Input: dimensioned drawing with shaded views. Units: mm. Origin: part minimum x, y, z. Give positions to 0.01 mm unless a question says otherwise; leave off trailing zeros. Write each loop counter-clockwise with the first axis right and the second up, starting at its lowest first coordinate (ties: lowest second). Pieces come first, ordered by that corner, then holes.
Q1. Section B-B (z = 25). Return the cut outline in (x, y), plus the area to 3 significant figures.
Q2. Line query: line 1 (Z direction, x = 190, y = 1.6); line 2 (X direction, y = 1.65, z = 16); line 3 (Z direction, x = 127, y = 1.45). Output: solid intervals per line, ascending.
Q3. Pin query (flat end, axial travel): pin 1 Ø2.5 at (x, z) = (160, 21.25) entering from -Y. Return the tip coordinate at first contact, or that it passes through.
Q4. Section A-A (y = 0.8). Return the cut outline in (x, z).
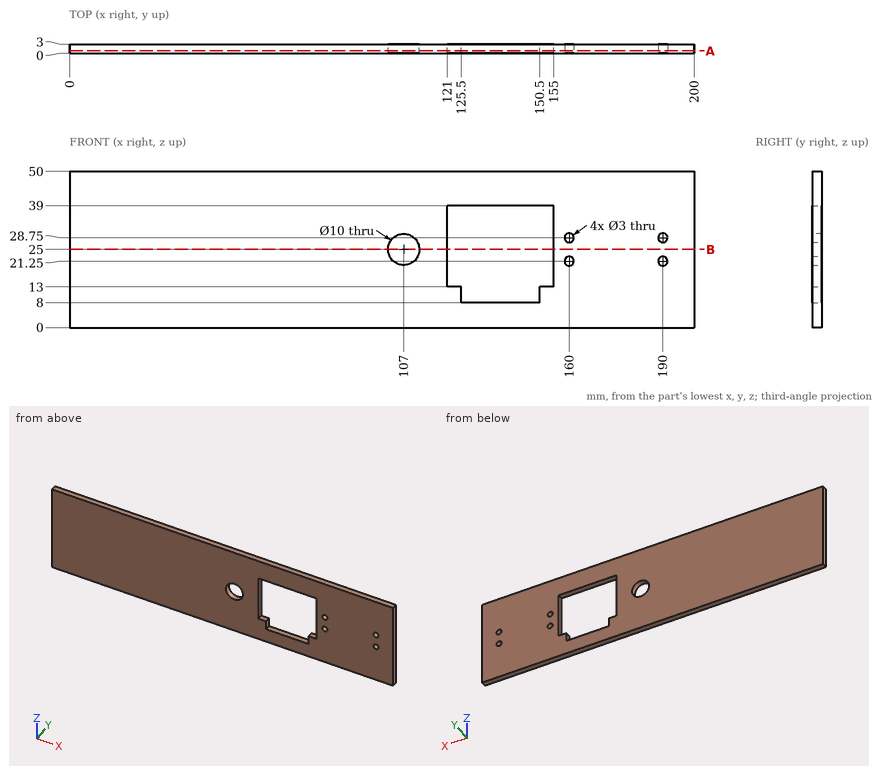
Computed:
1. outline: (0, 0) - (102, 0) - (102, 3) - (0, 3) - close; (112, 0) - (121, 0) - (121, 3) - (112, 3) - close; (155, 0) - (200, 0) - (200, 3) - (155, 3) - close
1. area: 468 mm2
2. line 1: z = 0 to 19.75, 22.75 to 27.25, 30.25 to 50
2. line 2: x = 0 to 121, 155 to 200
2. line 3: z = 0 to 8, 39 to 50
3. pin 1: passes through
4. outline: (0, 0) - (200, 0) - (200, 50) - (0, 50) - close; hole circle Ø10 at (107, 25); hole (121, 13) - (125.5, 13) - (125.5, 8) - (150.5, 8) - (150.5, 13) - (155, 13) - (155, 39) - (121, 39) - close; hole circle Ø3 at (160, 21.25); hole circle Ø3 at (160, 28.75); hole circle Ø3 at (190, 21.25); hole circle Ø3 at (190, 28.75)
